Autodesk Inventor part; units mm, degrees
ref_plane "YZ Plane" through (0, 0, 0) normal (1, 0, 0) x (0, 1, 0)
ref_plane "XZ Plane" through (0, 0, 0) normal (0, 1, 0) x (-1, 0, 0)
ref_plane "XY Plane" through (0, 0, 0) normal (0, 0, 1) x (1, 0, 0)
sketch "Sketch1" plane through (0, 0, 0) normal (1, 0, 0) x (0, 1, 0)
  line L0 (7.7549, 10.0308) -> (1.4049, 10.0308)
  line L1 (-1.7701, 6.8558) -> (-1.7701, 0.5058)
  line L2 (1.4049, -2.6692) -> (7.7549, -2.6692)
  line L3 (10.9299, 0.5058) -> (10.9299, 6.8558)
  arc A0 (10.9299, 6.8558) -> (7.7549, 10.0308) centre (7.7549, 6.8558) ccw
  arc A1 (7.7549, -2.6692) -> (10.9299, 0.5058) centre (7.7549, 0.5058) ccw
  arc A2 (-1.7701, 0.5058) -> (1.4049, -2.6692) centre (1.4049, 0.5058) ccw
  arc A3 (1.4049, 10.0308) -> (-1.7701, 6.8558) centre (1.4049, 6.8558) ccw
  point P0 (0, 0)
  point P1 (10.9299, 10.0308)
  point P2 (-1.7701, -2.6692)
  point P3 (-1.7701, 10.0308)
  dimension "d0" = 12.7
  dimension "d1" = 12.7
  dimension "d2" = 3.175
extrude "Extrusion1" add sketch "Sketch1" along normal blind 241.3
sketch "Sketch2" plane through (0, 10.9299, 6.8558) normal (0, 1, 0) x (1, 0, 0)
  line L0 (0, -22.225) -> (15.24, -22.225)
  line L1 (15.24, -22.225) -> (15.24, 28.575)
  line L2 (15.24, 28.575) -> (0, 28.575)
  line L3 (0, 28.575) -> (0, -22.225)
  line L4 (0, -3.175) -> (241.3, -3.175)
  line L5 (0, 9.525) -> (241.3, 9.525)
  line L6 (226.06, -22.225) -> (241.3, -22.225)
  line L7 (241.3, -22.225) -> (241.3, 28.575)
  line L8 (241.3, 28.575) -> (226.06, 28.575)
  line L9 (226.06, 28.575) -> (226.06, -22.225)
  line L10 (241.3, 6.35) -> (241.3, 0)
  point P0 (0, 6.8558)
  dimension "d5" = 19.05
  dimension "d6" = 19.05
  dimension "d7" = 15.24
  dimension "d8" = 0
  dimension "d9" = 19.05
  dimension "d10" = 19.05
  dimension "d11" = 15.24
extrude "Extrusion2" add sketch "Sketch2" along normal blind 38.1 contours L3 L4 L1 L0 | L3 L5 L1 L4 | L3 L2 L1 L5 | L9 L5 L7 L4 | L4 L7 L6 L9 | L9 L8 L7 L5
sketch "Sketch4" plane through (241.3, 0, 0) normal (1, 0, 0) x (0, 0, -1)
  line L0 (-29.0808, 10.9299) -> (-6.8558, 10.9299)
  line L1 (-0.5058, 10.9299) -> (21.7192, 10.9299)
  line L2 (-6.8558, -1.7701) -> (-0.5058, -1.7701)
  line L3 (-6.8558, -1.7701) -> (-29.0808, 10.9299)
  line L4 (-6.8558, -1.7701) -> (-0.5058, -1.7701)
  line L5 (-0.5058, -1.7701) -> (21.7192, 10.9299)
  line L6 (-0.5058, -1.7701) -> (-6.8558, -1.7701)
  line L7 (-6.8558, 10.9299) -> (-29.0808, 10.9299)
  line L8 (21.7192, 10.9299) -> (-29.0808, 10.9299)
  point P0 (0, 0)
extrude "Extrusion3" add sketch "Sketch4" against normal blind 12.7
sketch "Sketch3" plane through (0, 49.0299, 6.8558) normal (0, 1, 0) x (1, 0, 0)
  line L0 (0, -22.225) -> (15.24, -22.225)
  line L1 (0, 28.575) -> (0, -22.225)
  line L2 (241.3, -22.225) -> (241.3, 28.575)
  line L3 (241.3, 28.575) -> (226.06, 28.575)
  line L4 (226.06, -22.225) -> (241.3, -22.225)
  point P0 (0, 6.8558)
  point P1 (6.35, -9.525)
  point P2 (6.35, 15.875)
  point P3 (234.95, -9.525)
  point P4 (234.95, 15.875)
  dimension "d14" = 25.4
  dimension "d15" = 12.7
  dimension "d16" = 0
  dimension "d17" = 6.35
  dimension "d18" = 0
  dimension "d19" = 6.35
  dimension "d20" = 12.7
  dimension "d21" = 12.7
hole "Hole1" at (6.35, 49.0299, 16.3808) at (6.35, 49.0299, -9.0192) at (234.95, 49.0299, 16.3808) at (234.95, 49.0299, -9.0192) direction (0, -1, 0) diameter 4.4958 depth 25.4 tip angle 118
sketch "Sketch5" plane through (0, 0, 0) normal (-1, 0, 0) x (0, 0, 1)
  line L0 (6.8558, -1.7701) -> (0.5058, -1.7701)
  line L1 (6.8558, 10.9299) -> (29.0808, 10.9299)
  line L2 (-21.7192, 10.9299) -> (0.5058, 10.9299)
  line L3 (-21.7192, 10.9299) -> (-2.2296, -0.2071)
  line L4 (29.0808, 10.9299) -> (-21.7192, 10.9299)
  line L5 (-21.7192, 10.9299) -> (0.5058, -1.7701)
  line L6 (6.8558, -1.7701) -> (0.5058, -1.7701)
  line L7 (29.0808, 10.9299) -> (29.0808, 49.0299)
  line L8 (6.8558, -1.7701) -> (29.0808, 10.9299)
  point P0 (0, 0)
extrude "Extrusion4" add sketch "Sketch5" against normal blind 12.7
sketch "Sketch6" plane through (0, 49.0299, 6.8558) normal (0, 1, 0) x (1, 0, 0)
  circle A0 centre (6.35, -9.525) radius 2.2479
  circle A1 centre (6.35, 15.875) radius 2.2479
  circle A2 centre (234.95, -9.525) radius 2.2479
  circle A3 centre (234.95, 15.875) radius 2.2479
  circle A4 centre (234.95, -9.525) radius 2.2479
  point P0 (0, 6.8558)
hole "Hole2" at (234.95, 49.0299, 16.3808) at (234.95, 49.0299, -9.0192) at (6.35, 49.0299, -9.0192) at (6.35, 49.0299, 16.3808) direction (0, -1, 0) diameter 4.4958 end through all
sketch "Sketch7" plane through (0, -1.7701, 0.5058) normal (0, -1, 0) x (1, 0, 0)
  circle A0 centre (6.35, -9.525) radius 2.2479
  circle A1 centre (6.35, 15.875) radius 2.2479
  circle A2 centre (234.95, 15.875) radius 2.2479
  circle A3 centre (234.95, -9.525) radius 2.2479
  circle A4 centre (234.95, -9.525) radius 5.08
  circle A5 centre (234.95, 15.875) radius 5.08
  circle A6 centre (6.35, -9.525) radius 5.08
  circle A7 centre (6.35, 15.875) radius 5.08
  point P0 (0, -0.5058)
  dimension "d40" = 10.16
  dimension "d41" = 10.16
  dimension "d42" = 10.16
  dimension "d43" = 10.16
extrude "Extrusion5" cut sketch "Sketch7" against normal blind 12.7
sketch "Sketch8" plane through (0, 49.0299, 6.8558) normal (0, 1, 0) x (1, 0, 0)
  line L0 (261.8512, -57.5381) -> (-18.787, -57.5381)
  line L1 (-18.787, -57.5381) -> (-18.787, -19.685)
  line L2 (-18.787, -19.685) -> (261.8512, -19.685)
  line L3 (261.8512, -19.685) -> (261.8512, -57.5381)
  line L4 (261.8512, 26.035) -> (-15.1591, 26.035)
  line L5 (-15.1591, 26.035) -> (-15.1591, 48.4462)
  line L6 (-15.1591, 48.4462) -> (261.8512, 48.4462)
  line L7 (261.8512, 48.4462) -> (261.8512, 26.035)
  line L8 (226.06, -22.225) -> (241.3, -22.225)
  line L9 (241.3, 28.575) -> (226.06, 28.575)
  point P0 (0, 6.8558)
  dimension "d46" = 2.54
  dimension "d47" = 2.54
extrude "Extrusion6" cut sketch "Sketch8" against normal blind 71.4375
properties part number "Handle"
CAD build for the part. Positions are in the model's coordinates, mm. A direction names the side the tool comes from. Round coordinates to 2 decimals unless told otherwise and drop trailing zeros. Loops run counter-clockwise (first coordinate to the right, second up) from the corner with the lowest first, then second, coordinate; pieces in that order, holes last.
(1) Drop flat-ended pins along their axis: pin 1 (8 mm diameter, centred on x = 234.95, z = 16.38, fed in from -Y); pin 2 (12.5 mm diameter, centred on y = 7.5, z = 21, fed in from -X); pin 3 (8 mm diameter, centred on x = 7.5, z = -7, fed in from -Y); pin 4 (4 mm diameter, centred on x = 6.35, z = -9.02, fed in from +Y). Give the stop position or say it passes through.
(2) Cut at C-C (z = 24.5). Give the cut face in (x, y), plus the area to 3 significant figures.
(3) Which spindle directions (+Z, -Z, +X, -X, +Y, -Y) get a long thin tool onto all of the face, cutting with end or side? Do faces 1 (the cylindrical face through (234.289, 6.904, -3.982)), 2 (the flat face through (0, 23, 4)), 3 (the flat face through (226.06, 30, 3)). Say none if no direction does.
(4) Cut at A-A (y = 28). Give the cut face in (x, z), plus the area to 3 significant figures.
(5) Cut at B-B (x = 6.35). Give the cut face in (y, z) (3 decimals), plus the area to 3 significant figures.
(6) Cut at D-D (x = 135.5). Give the cut face in (y, z) (3 decimals).
(7) Wall check: line 1 along Z through (x, y) = (6, 39); line 2 along Z through (x, y) = (234.95, 37); line 3 along X through (y, z) = (41, -16). Give the ranges that are in metal, low to high.
Findings below:
1. pin 1: stops at y = 10.93
1. pin 2: stops at x = 0
1. pin 3: stops at y = 0.23
1. pin 4: passes through
2. outline: (0, 8.31) - (12.7, 8.31) - (12.7, 10.93) - (15.24, 10.93) - (15.24, 49.03) - (0, 49.03) - close; (226.06, 10.93) - (228.6, 10.93) - (228.6, 8.31) - (241.3, 8.31) - (241.3, 49.03) - (226.06, 49.03) - close
2. area: 1,230 mm2
3. face 1: -Y
3. face 2: +Z, -Z, -X, +Y, -Y
3. face 3: +Z, -Z, +Y
4. outline: (0, -19.18) - (15.24, -19.18) - (15.24, 26.54) - (0, 26.54) - close; (226.06, -19.18) - (241.3, -19.18) - (241.3, 26.54) - (226.06, 26.54) - close; hole circle Ø4.5 at (6.35, -9.02); hole circle Ø4.5 at (6.35, 16.38); hole circle Ø4.5 at (234.95, -9.02); hole circle Ø4.5 at (234.95, 16.38)
4. area: 1,330 mm2
5. outline: (-1.77, 0.506) arc R3.175 ccw to (-0.207, -2.23) - (0.77, -3.939) - (10.93, -3.939) - (10.93, -6.771) - (49.03, -6.771) - (49.03, 14.133) - (10.93, 14.133) - (10.93, 11.301) - (0.77, 11.301) - (-0.207, 9.591) arc R3.175 ccw to (-1.77, 6.856) - close; (6.576, -14.099) - (9.478, -19.179) - (49.03, -19.179) - (49.03, -11.267) - (10.93, -11.267) - (10.93, -14.099) - close; (6.576, 21.461) - (10.93, 21.461) - (10.93, 18.629) - (49.03, 18.629) - (49.03, 26.541) - (9.478, 26.541) - close
5. area: 1,610 mm2
6. outline: (-1.77, 0.506) arc R3.175 ccw to (1.405, -2.669) - (7.755, -2.669) arc R3.175 ccw to (10.93, 0.506) - (10.93, 6.856) arc R3.175 ccw to (7.755, 10.031) - (1.405, 10.031) arc R3.175 ccw to (-1.77, 6.856) - close
7. line 1: z = -19.18 to -11.24, -6.8 to 14.16, 18.6 to 26.54
7. line 2: z = -19.18 to -11.27, -6.77 to 14.13, 18.63 to 26.54
7. line 3: x = 0 to 15.24, 226.06 to 241.3
